The model under review builds one solid part; all positions refer to its coordinate system, in mm. A direction names the side the tool comes from. Coordinates: 2 decimals unless noted, no trailing zeros. Loops run counter-clockwise (first coordinate to the right, second up) from the corner with the lowest first, then second, coordinate; pieces in that order, holes last. Notation, with made-up numbers: M 6,44 L 24,44 A30 cw 24,67 Z; hole C -31,58 d4. An arc over 180 degrees is marked long. Use CSV: the item, a comma, the result in double quotes. Start each with the question number.
1. Add section C-C, the plane z = -19. Write out the cut boundary in (x, y), then the cut area to 3 significant figures.
2. Add section B-B, the plane x = 2. State how many separate pieces and enclosed holes the cut face has, then the cut area to 3 significant figures.
3. Draft analysis for pull direction X (two halves, no side actions). For faces 1 (the flat face through (21, -23.8, 1)), 2 (the flat face through (0, -15, 0)), 3 (the cylindrical face through (-6, -21, 0)), state which applies: +X half, -X half, draft (parallel to the pull), parting line (faces both ways), or undercut.
4. Clearance check with flat-ended pins moving along their axes: P1, Ø1.1, axis at y = -24.5, z = -16, coming from the -X side; P2, Ø1.1, axis at x = -9.5, y = -24, coming from the -Z side; P3, Ø4.5, axis at x = -14.5, z = -0.5, coming from the +Y side; P4, Ø3.5, axis at x = 0, z = 0.5, coming from the +Y side. State where each tip first meets the part, or that it passes through.
5. Add section D-D, the plane x = 17. Write out the cut boundary in (y, z), then the cut area to 3 significant figures.
6. Add section A-A, the plane y = -21.5. Write out the cut boundary in (x, z).
7. Tool access review of faces 4 (the flat face through (0, -17, 0)), 5 (the flat face through (2, -24.8, 6)), 6 (the flat face through (0, -23.8, 16)), 7 (the cylindrical face through (-0.75, -7.76, 5.7)): name each direction out of +Z, -Z, +X, -X, +Y, -Y from which nothing blocks a thin tool from reaching the whole face with its end or side.
8. For L1, parallel to Z at x = 0, y = -6; L2, parallel to Y at x = 18.5, z = -3.5; L3, parallel to Z at x = 0, y = -19, list the stretches that pass through material, from the lowest coordinate up.
from build123d import *

# Parameters (mm, degrees)
F0_R      = 7.75
F0_R_2    = 5.75
F1_DEPTH  = 7.75
F2_R      = 7.74999
F3_DEPTH  = 15
F4_DEPTH  = 5
F6_R      = 7.75
F6_R_2    = 6
F7_DEPTH  = 9.8
F6_R_3    = 5.75
F8_DEPTH  = 2
F10_DEPTH = 1


# Not quite as in the source:
# - a fillet or chamfer that OpenCascade refuses, or shapes differently, is made with other operations: its cross-section is extruded or revolved along the edge and cut away or added
# - a fillet or chamfer is up to 0.001 mm smaller than in the source, because OpenCascade refuses the exact size


with BuildPart() as f1:
    # F0 (on Front) → F1 (new body)
    with BuildSketch(Plane.XZ):
        Circle(F0_R)
        Circle(F0_R_2, mode=Mode.SUBTRACT)
        Circle(F0_R_2)
    extrude(amount=-F1_DEPTH)

    # F2 (radius 7.75 in the source; OpenCascade refuses exactly that, so slightly less here)
    f2_edges = [f1.edges().sort_by_distance(p)[0] for p in [
        (-7.75, 7.75, 0),
    ]]
    fillet(f2_edges, radius=F2_R)

    # F0 (on Front) → F3 (join)
    with BuildSketch(Plane.XZ):
        Circle(F0_R)
        Circle(F0_R_2, mode=Mode.SUBTRACT)
    extrude(amount=F3_DEPTH)

    # F0 (on Front) → F4 (cut)
    with BuildSketch(Plane.XZ):
        Circle(F0_R_2)
    extrude(amount=-F4_DEPTH, mode=Mode.SUBTRACT)

    # F5: fillet of radius 5.75 on 1 edges, made by hand

    # F5_s1 → F5_t2 (revolve)
    with BuildSketch(Plane.XY):
        with BuildLine():
            ThreePointArc((5.7501, -0.7499), (4.0659639918, 3.3159639918), (0.0001, 5.0001))
            Line((0.0001, 5.0001), (0.0001, 5.1151))
            ThreePointArc((0.0001, 5.1151), (2.87505, 5.115), (5.75, 5.115))
            Line((5.75, 5.115), (5.865, 5))
            ThreePointArc((5.865, 5), (5.865, 2.12505), (5.8651, -0.7499))
            Line((5.8651, -0.7499), (5.7501, -0.7499))
        make_face()
    revolve(axis=Axis((0, 5, 0), (0, -1, 0)))

    # F6 (on face) → F7 (join)
    with BuildSketch(Plane.XZ.offset(15)):
        Circle(F6_R)
        Circle(F6_R_2, mode=Mode.SUBTRACT)
    extrude(amount=F7_DEPTH)

    # F6 (on face) → F8 (join)
    with BuildSketch(Plane.XZ.offset(15)):
        Circle(F6_R_2)
        Circle(F6_R_3, mode=Mode.SUBTRACT)
        Circle(F6_R_3)
    extrude(amount=F8_DEPTH)

    # F9 (on face) → F10 (join)
    with BuildSketch(Plane.XZ.offset(24.8)):
        with BuildLine():
            ThreePointArc((-7.6053065566, -1.4905744465), (-7.7379420075, -0.4321498454), (-7.7239859171, 0.6344616239))
            Line((-7.7239859171, 0.6344616239), (-11.2089226057, 0.6344616239))
            Line((-11.2089226057, 0.6344616239), (-11.2089226057, 7.51422951))
            Line((-11.2089226057, 7.51422951), (-24.211389944, 7.51422951))
            Line((-24.211389944, 7.51422951), (-24.211389944, -6.8491166458))
            Line((-24.211389944, -6.8491166458), (-11.4740878344, -6.8491166458))
            Line((-11.4740878344, -6.8491166458), (-11.4740878344, -1.4905744465))
            Line((-11.4740878344, -1.4905744465), (-7.6053065566, -1.4905744465))
        make_face()
        with BuildLine():
            ThreePointArc((-1.3181141258, 7.6370855142), (-0.2358353441, 7.7464108909), (0.8510895829, 7.7031257631))
            Line((0.8510895829, 7.7031257631), (0.8510895829, 10.0341412146))
            Line((0.8510895829, 10.0341412146), (8.7516037747, 10.0341412146))
            Line((8.7516037747, 10.0341412146), (8.7516037747, 23.6629825085))
            Line((8.7516037747, 23.6629825085), (-8.5408838931, 23.6629825085))
            Line((-8.5408838931, 23.6629825085), (-8.5408838931, 10.2677652612))
            Line((-8.5408838931, 10.2677652612), (-8.5408838931, 10.0341412146))
            Line((-8.5408838931, 10.0341412146), (-1.3181141258, 10.0341412146))
            Line((-1.3181141258, 10.0341412146), (-1.3181141258, 7.6370855142))
        make_face()
        with BuildLine():
            Line((13.07656436, 0.9255647358), (7.6945324692, 0.9255647358))
            ThreePointArc((7.6945324692, 0.9255647358), (7.7361206892, 0.463612642), (7.75, 0))
            ThreePointArc((7.75, 0), (7.7293938157, -0.5647753903), (7.6676848409, -1.1265474604))
            Line((7.6676848409, -1.1265474604), (13.6271854863, -1.1265474604))
            Line((13.6271854863, -1.1265474604), (13.6271854863, -7.3085245676))
            Line((13.6271854863, -7.3085245676), (29.0946420282, -7.3085245676))
            Line((29.0946420282, -7.3085245676), (29.0946420282, 8.8346945122))
            Line((29.0946420282, 8.8346945122), (13.07656436, 8.8346945122))
            Line((13.07656436, 8.8346945122), (13.07656436, 0.9255647358))
        make_face()
        with BuildLine():
            Line((1.256284304, -11.5922550619), (1.256284304, -7.6474995749))
            ThreePointArc((1.256284304, -7.6474995749), (0.1659608629, -7.748222828), (-0.9276754413, -7.6942782817))
            Line((-0.9276754413, -7.6942782817), (-0.9276754413, -11.5922550619))
            Line((-0.9276754413, -11.5922550619), (-8.4876073524, -11.5922550619))
            Line((-8.4876073524, -11.5922550619), (-8.4876073524, -23.2104603201))
            Line((-8.4876073524, -23.2104603201), (9.6937846392, -23.2104603201))
            Line((9.6937846392, -23.2104603201), (9.6937846392, -11.5922550619))
            Line((9.6937846392, -11.5922550619), (1.256284304, -11.5922550619))
        make_face()
    extrude(amount=-F10_DEPTH)


solid = f1.part
Computed:
1,outline,"M -8.49,-24.8 L 9.69,-24.8 L 9.69,-23.8 L -8.49,-23.8 Z"
1,area,"18.2 mm^2"
2,separate pieces,"3"
2,enclosed holes,"1"
2,area,"197 mm^2"
3,face 1,"draft"
3,face 2,"undercut"
3,face 3,"undercut"
4,P1,"stops at x = -8.49"
4,P2,"stops at z = -1.49"
4,P3,"stops at y = -23.8"
4,P4,"stops at y = 7.75"
5,outline,"M -24.8,-7.31 L -23.8,-7.31 L -23.8,8.83 L -24.8,8.83 Z"
5,area,"16.1 mm^2"
6,outline,"C 0,0 d15.5; hole C 0,0 d12"
7,face 4,"-Y"
7,face 5,"+Z, -Z, +X, -X, -Y"
7,face 6,"+Z, +X, -X, +Y"
7,face 7,"none"
8,L1,"z = -7.75 to -5.75, 5.75 to 7.75"
8,L2,"y = -24.8 to -23.8"
8,L3,"z = -7.75 to -6, 6 to 7.75"
